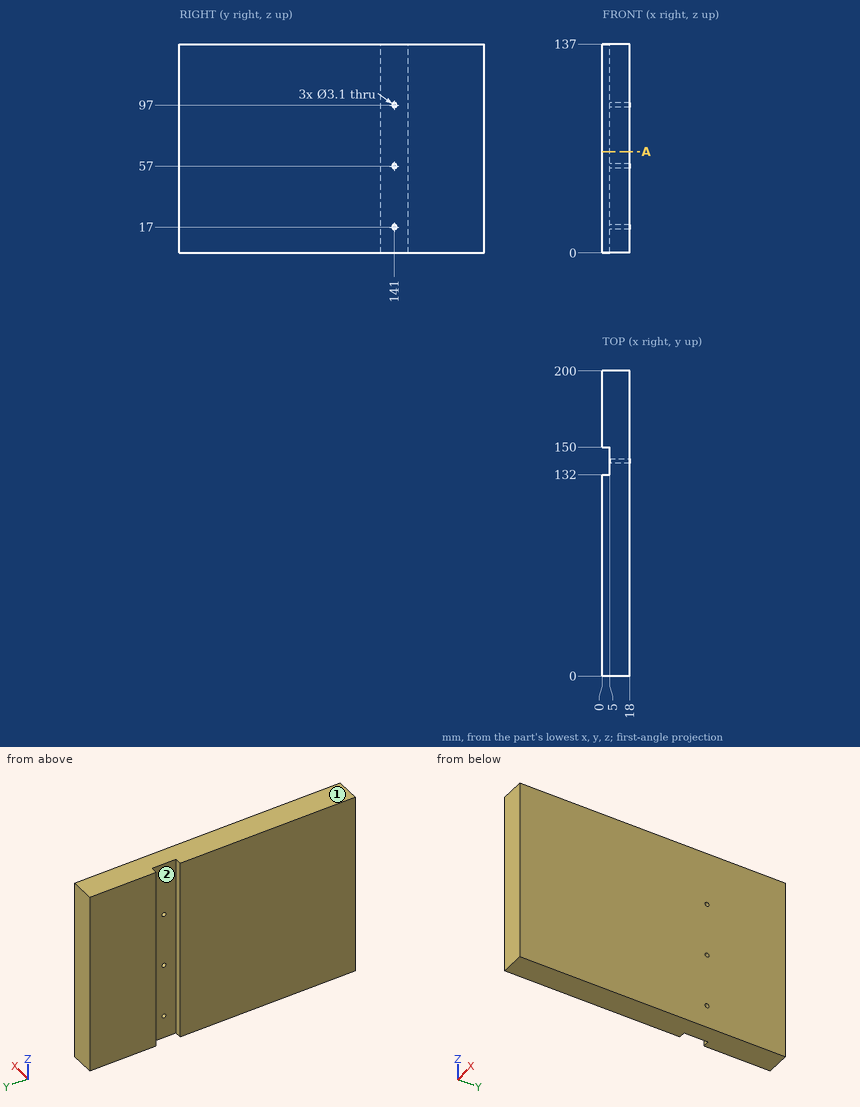
Verification items for this drawing (mm, ordinates from the low corner). Coordinates: 2 decimals unless noted, no trailing zeros. Loops run counter-clockwise (first coordinate to the right, second up) from the corner with the lowest first, then second, coordinate; pieces in that order, holes last. Notation, with made-up numbers: (63, 89) - (86, 89) arc R25 cw to (86, 122) - close; hole circle Ø3 at (19, -18.5). An arc over 180 degrees is marked (long way). One line per item, written item: value. Start each with the question number.
(1) Mould release check, pull along Y, two halves, no side actions. Record for the marked faces 1 and 2: released by +Y, released by -Y, zero draft, split by the parting line, or undercut.
(2) Material ranges on line 1 (Y direction, x = 1.25, z = 72); line 2 (X direction, y = 148, z = 118.5); line 3 (Y direction, x = 11, z = 58), recorded low to high. Write a range as [from, to].
(3) Depth check by flat-ended pin: P1, Ø9, axis at y = 137.5, z = 79.5, coming from the -X side. Enter the tip coordinate at first touch or a pass-through.
(4) Cross-section at A-A on z = 66.5. Enter the section's corners in (x, y).
Results below:
1. face 1: zero draft
1. face 2: undercut
2. line 1: y = [0, 132], [150, 200]
2. line 2: x = [5, 18]
2. line 3: y = [0, 139.82], [142.18, 200]
3. P1: stops at x = 5
4. outline: (0, 0) - (18, 0) - (18, 200) - (0, 200) - (0, 150) - (5, 150) - (5, 132) - (0, 132) - close
